from build123d import *

# Parameters (mm, degrees)
SKETCH1_W           = 30
SKETCH1_H           = 30
BOSS_EXTRUDE1_DEPTH = 140
SKETCH2_W           = 20
SKETCH2_H           = 20
BOSS_EXTRUDE2_DEPTH = 5
SKETCH3_W           = 20.5
SKETCH3_H           = 20.5
CUT_EXTRUDE1_DEPTH  = 10


with BuildPart() as part:
    # Sketch1 → Boss-Extrude1 (new body)
    with BuildSketch(Plane.XY):
        Rectangle(SKETCH1_W, SKETCH1_H)
    extrude(amount=BOSS_EXTRUDE1_DEPTH)

    # Sketch2 → Boss-Extrude2 (add)
    with BuildSketch(Plane.XY):
        Rectangle(SKETCH2_W, SKETCH2_H)
    extrude(amount=-BOSS_EXTRUDE2_DEPTH)

    # Sketch3 → Cut-Extrude1 (cut)
    with BuildSketch(Plane.XY.offset(140)):
        Rectangle(SKETCH3_W, SKETCH3_H)
    extrude(amount=-CUT_EXTRUDE1_DEPTH, mode=Mode.SUBTRACT)


solid = part.part
Geometry: final body of the model. Coordinates: model frame, mm. A direction names the side the tool comes from. Give positions to 0.01 mm unless a question says otherwise; leave off trailing zeros. Loops run counter-clockwise (first coordinate to the right, second up) from the corner with the lowest first, then second, coordinate; pieces in that order, holes last. Notation, with made-up numbers: M -28,21.25 L 28,21.25 A12 ccw 28,43.25 Z; hole C -16.75,-28 d6. An arc over 180 degrees is marked long. Put each result on its own line as item: value. Start each with the question number.
1) Contact query for flat-ended pins moving along their axis: pin 1 (2 mm diameter, centred on x = -8.5, y = 2.5, fed in from +Z); pin 2 (5.5 mm diameter, centred on y = -2, z = -2.5, fed in from -X); pin 3 (4 mm diameter, centred on x = -1.5, z = -3, fed in from +Y). Output: stop coordinate, or through.
2) Cut plane A-A (x = 7.5). Output: boundary loops of the cut face in (y, z), then the cut area to 4 significant figures.
3) Cut plane C-C (x = -13). Output: boundary loops of the cut face in (y, z).
4) Pull-direction query (Y, two-part tool) for faces 6 (the flat face through (0, 10, -2)), 7 (the flat face through (15, 0, 69)), 8 (the flat face through (0, -10.25, 135)); classes: pulls with the +Y half, pulls with the -Y half, needs draft (parallel to the pull), parting line crosses it, or undercut.
5) Ray query, line 1 along Z through (x, y) = (9.75, -2.75); line 2 along Z through (x, y) = (-7.75, 13.5); line 3 along X through (y, z) = (-9.75, 131). Return the intervals inside material, ascending.
6) Access query for faces 1 (the flat face through (0, 15, 69)), 2 (the flat face through (10.25, 0, 135)), 3 (the flat face through (10, 0, -2)), 4 (the flat face through (0, -10, -2)), 5 (the flat face through (-10, 0, -2)). Directions: +Z, -Z, +X, -X, +Y, -Y. A direction counts if a zero-diameter tool reaches every point of the face in a straight line with its end or side. Return the directions, or none.
Verdict:
1. pin 1: z = 130
1. pin 2: x = -15
1. pin 3: y = 10
2. outline: M -15,0 L -10,0 L -10,-5 L 10,-5 L 10,0 L 15,0 L 15,140 L 10.25,140 L 10.25,130 L -10.25,130 L -10.25,140 L -15,140 Z
2. area: 4,095 mm2
3. outline: M -15,0 L 15,0 L 15,140 L -15,140 Z
4. face 6: pulls with the +Y half
4. face 7: needs draft
4. face 8: undercut
5. line 1: -5 to 130
5. line 2: 0 to 140
5. line 3: -15 to -10.25, 10.25 to 15
6. face 1: +Z, -Z, +X, -X, +Y
6. face 2: +Z
6. face 3: -Z, +X, +Y, -Y
6. face 4: -Z, +X, -X, -Y
6. face 5: -Z, -X, +Y, -Y
